from build123d import *

# Parameters (mm, degrees)
BOSS_EXTRUDE1_DEPTH = 5
SKETCH10_R          = 19.05
SKETCH10_R_2        = 2.5
SKETCH10_R_3        = 25
CUT_EXTRUDE7_DEPTH  = 6
SKETCH11_R          = 31
CUT_EXTRUDE8_DEPTH  = 2
CUT_EXTRUDE9_DEPTH  = 6


with BuildPart() as part:
    # Sketch1 → Boss-Extrude1 (new body)
    with BuildSketch(Plane(origin=(0, 0, 0), x_dir=(1, 0, 0), z_dir=(0, 1, 0))):
        with BuildLine():
            Line((15.254575611, 35.990242765), (15.254575611, 44.990242765))
            ThreePointArc((15.254575611, 44.990242765), (13.790109517, 48.525776671), (10.254575611, 49.990242765))
            Line((10.254575611, 49.990242765), (-50.745424389, 49.990242765))
            ThreePointArc((-50.745424389, 49.990242765), (-99.757685432, 0), (-50.745424389, -49.990242765))
            Line((-50.745424389, -49.990242765), (10.254575611, -49.990242765))
            ThreePointArc((10.254575611, -49.990242765), (13.790109517, -48.525776671), (15.254575611, -44.990242765))
            Line((15.254575611, -44.990242765), (15.254575611, -35.990242765))
            ThreePointArc((15.254575611, -35.990242765), (16.133255268, -33.868922422), (18.254575611, -32.990242765))
            Line((18.254575611, -32.990242765), (22.711934924, -32.990242765))
            ThreePointArc((22.711934924, -32.990242765), (23.859985221, -33.218604168), (24.833255268, -33.868922422))
            Line((24.833255268, -33.868922422), (40.954575611, -49.990242765))
            Line((40.954575611, -49.990242765), (50.745424389, -49.990242765))
            Line((50.745424389, -49.990242765), (94.067824265, -49.990242765))
            ThreePointArc((94.067824265, -49.990242765), (96.567824265, -50.660115747), (98.397951284, -52.490242765))
            Line((98.397951284, -52.490242765), (114.280717029, -80))
            Line((114.280717029, -80), (134.280717029, -80))
            Line((134.280717029, -80), (134.280717029, 80))
            Line((134.280717029, 80), (114.280717029, 80))
            Line((114.280717029, 80), (98.397951284, 52.490242765))
            ThreePointArc((98.397951284, 52.490242765), (96.567824265, 50.660115747), (94.067824265, 49.990242765))
            Line((94.067824265, 49.990242765), (50.745424389, 49.990242765))
            Line((50.745424389, 49.990242765), (40.954575611, 49.990242765))
            Line((40.954575611, 49.990242765), (24.833255268, 33.868922422))
            ThreePointArc((24.833255268, 33.868922422), (23.859985221, 33.218604168), (22.711934924, 32.990242765))
            Line((22.711934924, 32.990242765), (18.254575611, 32.990242765))
            ThreePointArc((18.254575611, 32.990242765), (16.133255268, 33.868922422), (15.254575611, 35.990242765))
        make_face()
    extrude(amount=BOSS_EXTRUDE1_DEPTH)

    # Sketch10 → Cut-Extrude7 (cut, through all)
    with BuildSketch(Plane(origin=(0, 5, 0), x_dir=(1, 0, 0), z_dir=(0, 1, 0))):
        with Locations((79.280717029, 0)):
            Circle(SKETCH10_R)
        with Locations((55.710717029, 23.57)):
            Circle(SKETCH10_R_2)
        with Locations((102.850717029, 23.57)):
            Circle(SKETCH10_R_2)
        with Locations((102.850717029, -23.57)):
            Circle(SKETCH10_R_2)
        with Locations((55.710717029, -23.57)):
            Circle(SKETCH10_R_2)
        with Locations((-49.757685432, 0)):
            Circle(SKETCH10_R_3)
    extrude(amount=-CUT_EXTRUDE7_DEPTH, mode=Mode.SUBTRACT)

    # Sketch11 → Cut-Extrude8 (cut)
    with BuildSketch(Plane.XZ):
        with Locations((-49.757685432, 0)):
            Circle(SKETCH11_R)
    extrude(amount=-CUT_EXTRUDE8_DEPTH, mode=Mode.SUBTRACT)

    # Sketch12 → Cut-Extrude9 (cut, through all)
    with BuildSketch(Plane.XZ):
        with BuildLine():
            Line((-2.257685432, 37.5), (-2.257685432, 22.5))
            ThreePointArc((-2.257685432, 22.5), (0.242314568, 20), (2.742314568, 22.5))
            Line((2.742314568, 22.5), (2.742314568, 37.5))
            ThreePointArc((2.742314568, 37.5), (0.242314568, 40), (-2.257685432, 37.5))
        make_face()
    extrude(amount=-CUT_EXTRUDE9_DEPTH, mode=Mode.SUBTRACT)


solid = part.part
Here's how the part is built. I have some questions about the finished solid (model axes, mm). A direction names the side the tool comes from. Coordinates: 2 decimals unless noted, no trailing zeros. Write each loop counter-clockwise with the first axis right and the second up, starting at its lowest first coordinate (ties: lowest second). Pieces come first, ordered by that corner, then holes. Notation, with made-up numbers: (-28, 33) - (13, 33) arc R11 cw to (13, 38) - close; hole circle Ø5 at (-6, -30). An arc over 180 degrees is marked (long way). Use one line per item in the form item = value.
1) Suppose I cut it at A-A, the plane z = 10.5. Write out the boundary of the cut face in (x, y), plus the area to 3 significant figures.
Solved:
outline = (-98.64, 0) - (-78.93, 0) - (-78.93, 2) - (-72.45, 2) - (-72.45, 5) - (-98.64, 5) - close; (-27.07, 2) - (-20.59, 2) - (-20.59, 0) - (63.39, 0) - (63.39, 5) - (-27.07, 5) - close; (95.18, 0) - (134.28, 0) - (134.28, 5) - (95.18, 5) - close
area = 753 mm2
2) On a 3-axis mill with a long thin cutter (end or side, diameter ignored), from which of +Z, -Z, +X, -X, +Y, -Y can I reach the whole of each face in a straight line? I mean faces 1 (the flat face through (68, 2, -49.99)), 2 (the flat face through (15.255, 2, -40)), 3 (the flat face through (-21, 2, 49.99)). Say none if no direction works.
Solved:
face_1 = -Z, -X, +Y, -Y
face_2 = -Z, +Y, -Y
face_3 = +Z, -X, +Y, -Y
3) Thinking about a two-plate mould opening in Z: for faces 4 (the flat face through (42, 0, -1)), 5 (the flat face through (-71, 2, 14)), 6 (the flat face through (106.45, 2.46, -66.44)), which applies, released by +Z, released by -Z, zero draft, split by the parting line, or undercut?
Solved:
face_4 = zero draft
face_5 = undercut
face_6 = released by -Z
4) I need wall thicknesses on line 1 (X direction, y = 1.2, z = 23.57); line 2 (X direction, y = 0.3, z = -5.5); line 3 (Z direction, x = -51, y = 1.6). Which ranges of each line are inside material? Lowest first, please.
Solved:
line_1 = -93.85 to -69.89, -29.62 to -2.26, 2.74 to 53.21, 58.21 to 100.35, 105.35 to 134.28
line_2 = -99.45 to -80.27, -19.25 to 61.04, 97.52 to 134.28
line_3 = -49.98 to -30.98, 30.98 to 49.98
5) Suppose I cut it at D-D, the plane z = 55. Write out the boundary of the cut face in (x, y), plus the area to 3 significant figures.
Solved:
outline = (99.85, 0) - (134.28, 0) - (134.28, 5) - (99.85, 5) - close
area = 172 mm2
6) Suppose I cut it at B-B, the plane x = -38. Write out the boundary of the cut face in (y, z).
Solved:
outline = (0, -49.99) - (5, -49.99) - (5, -22.06) - (2, -22.06) - (2, -28.68) - (0, -28.68) - close; (0, 28.68) - (2, 28.68) - (2, 22.06) - (5, 22.06) - (5, 49.99) - (0, 49.99) - close
7) Suppose I cut it at C-C, the plane x = -70.5. Write out the boundary of the cut face in (y, z).
Solved:
outline = (0, -45.49) - (5, -45.49) - (5, -13.96) - (2, -13.96) - (2, -23.04) - (0, -23.04) - close; (0, 23.04) - (2, 23.04) - (2, 13.96) - (5, 13.96) - (5, 45.49) - (0, 45.49) - close
8) I'm going to push flat-ended pins straight in: P1, Ø2.5, axis at x = -18, y = 3.5, coming from the +Z side; P2, Ø2.5, axis at y = 2, z = 28, coming from the -X side; P3, Ø2, axis at y = 3, z = -28.5, coming from the -X side. Where does each tip first touch, or does it pass through?
Solved:
P1 = 49.99
P2 = -92
P3 = -91.52
